from build123d import *

# Parameters (mm, degrees)
ESQUISSE1_W             = 40
ESQUISSE1_H             = 40
BOSS_EXTRU_1_DEPTH      = 30
ENL_V_MAT_EXTRU_1_DEPTH = 30
ESQUISSE4_R             = 1.5
ENL_V_MAT_EXTRU_2_DEPTH = 41
ESQUISSE5_R             = 1.5
ENL_V_MAT_EXTRU_3_DEPTH = 41
ESQUISSE6_W             = 23
ESQUISSE6_H             = 27
ESQUISSE6_H_2           = 20.20636544
ESQUISSE6_H_3           = 20.206365439
BOSS_EXTRU_2_DEPTH      = 10
ESQUISSE7_R             = 3
ENL_V_MAT_EXTRU_4_DEPTH = 11.0000001


with BuildPart() as part:
    # Esquisse1 → Boss.-Extru.1 (new body)
    with BuildSketch(Plane.XY):
        with Locations((0, 559.576541314)):
            Rectangle(ESQUISSE1_W, ESQUISSE1_H)
        with BuildLine():
            Line((-10.025728158, 549.777097393), (9.970271386, 549.3770946))
            Line((9.970271386, 549.3770946), (9.998865294, 550.806494043))
            ThreePointArc((9.998865294, 550.806494043), (9.591165544, 551.864859717), (8.559153746, 552.335294236))
            Line((8.559153746, 552.335294236), (4.551996141, 552.495677906))
            ThreePointArc((4.551996141, 552.495677906), (2.508650242, 553.414808545), (1.671972976, 555.493277873))
            Line((1.671972976, 555.493277873), (1.671972976, 568.566900265))
            ThreePointArc((1.671972976, 568.566900265), (1.386115868, 569.266900215), (0.691973116, 569.566700242))
            Line((0.691973116, 569.566700242), (0.052575697, 569.579490838))
            ThreePointArc((0.052575697, 569.579490838), (-0.653001419, 569.307691005), (-0.966624431, 568.619683139))
            Line((-0.966624431, 568.619683139), (-1.489468376, 555.556519791))
            ThreePointArc((-1.489468376, 555.556519791), (-2.408599014, 553.513173892), (-4.487068342, 552.676496626))
            Line((-4.487068342, 552.676496626), (-8.497434284, 552.676496626))
            ThreePointArc((-8.497434284, 552.676496626), (-9.54743421, 552.247710964), (-9.99713425, 551.206496835))
            Line((-9.99713425, 551.206496835), (-10.025728158, 549.777097393))
        make_face(mode=Mode.SUBTRACT)
    extrude(amount=BOSS_EXTRU_1_DEPTH)

    # Esquisse3 → Enlèv. mat.-Extru.1 (cut)
    with BuildSketch(Plane.XY.offset(30)):
        with BuildLine():
            Line((0.701973186, 570.066600231), (0.062575767, 570.079390827))
            ThreePointArc((0.062575767, 570.079390827), (-0.995789907, 569.671691077), (-1.466224425, 568.639679279))
            Line((-1.466224425, 568.639679279), (-1.98906837, 555.57651593))
            ThreePointArc((-1.98906837, 555.57651593), (-2.755010569, 553.873727681), (-4.487068342, 553.176496626))
            Line((-4.487068342, 553.176496626), (-8.497434284, 553.176496626))
            ThreePointArc((-8.497434284, 553.176496626), (-9.897434185, 552.604782409), (-10.497034239, 551.216496905))
            Line((-10.497034239, 551.216496905), (-10.535628216, 549.287197474))
            Line((-10.535628216, 549.287197474), (10.460171305, 548.867194542))
            Line((10.460171305, 548.867194542), (10.498765283, 550.796493973))
            ThreePointArc((10.498765283, 550.796493973), (9.955165615, 552.207648206), (8.579149885, 552.83489423))
            Line((8.579149885, 552.83489423), (4.57199228, 552.995277901))
            ThreePointArc((4.57199228, 552.995277901), (2.869204031, 553.761220099), (2.171972976, 555.493277873))
            Line((2.171972976, 555.493277873), (2.171972976, 568.566900265))
            ThreePointArc((2.171972976, 568.566900265), (1.743187314, 569.61690019), (0.701973186, 570.066600231))
        make_face()
    extrude(amount=-ENL_V_MAT_EXTRU_1_DEPTH, mode=Mode.SUBTRACT)

    # Esquisse4 → Enlèv. mat.-Extru.2 (cut, through all)
    with BuildSketch(Plane.XZ.offset(-539.576541314)):
        with Locations(Location((-6.523433168, 24.203853726, 0), (0, 0, 270))):  # turned: the seam where the file's is
            Circle(ESQUISSE4_R)
        with Locations(Location((-6.523433168, 5.901559872, 0), (0, 0, 270))):  # turned: the seam where the file's is
            Circle(ESQUISSE4_R)
        with Locations((7.005369476, 5.612158233)):
            Circle(ESQUISSE4_R)
        with Locations((7.788039062, 23.897709596)):
            Circle(ESQUISSE4_R)
    extrude(amount=-ENL_V_MAT_EXTRU_2_DEPTH, mode=Mode.SUBTRACT)

    # Esquisse5 → Enlèv. mat.-Extru.3 (cut, through all)
    with BuildSketch(Plane.ZY.offset(20)):
        with Locations(Location((27.786828978, 562.049365696, 0), (0, 0, 270))):  # turned: the seam where the file's is
            Circle(ESQUISSE5_R)
        with Locations(Location((2.00094519, 562.049365696, 0), (0, 0, 270))):  # turned: the seam where the file's is
            Circle(ESQUISSE5_R)
    extrude(amount=-ENL_V_MAT_EXTRU_3_DEPTH, mode=Mode.SUBTRACT)

    # Esquisse6 → Boss.-Extru.2 (add)
    with BuildSketch(Plane(origin=(0, 0, 0), x_dir=(-1, 0, 0), z_dir=(0, 0, -1))):
        with Locations((-23.5, 581.076541314)):
            Rectangle(ESQUISSE6_W, ESQUISSE6_H)
        with Locations((22.166061681, 537.286666725)):
            Rectangle(ESQUISSE6_W, ESQUISSE6_H_2)
        with Locations((21.063566891, 581.241581079)):
            Rectangle(ESQUISSE6_W, ESQUISSE6_H)
        with Locations((-23.306010365, 536.648365215)):
            Rectangle(ESQUISSE6_W, ESQUISSE6_H_3)
    extrude(amount=-BOSS_EXTRU_2_DEPTH)

    # Esquisse7 → Enlèv. mat.-Extru.4 (cut, through all)
    with BuildSketch(Plane.XY.offset(10)):
        with Locations((-27.359707791, 589.516341352)):
            Circle(ESQUISSE7_R)
        with Locations((-27.359707791, 573.664786381)):
            Circle(ESQUISSE7_R)
        with Locations((-27.359707791, 541.773153337)):
            Circle(ESQUISSE7_R)
        with Locations((-27.359707791, 531.883070045)):
            Circle(ESQUISSE7_R)
        with Locations((-17.338422342, 531.883070045)):
            Circle(ESQUISSE7_R)
        with Locations((-17.338422342, 589.516341352)):
            Circle(ESQUISSE7_R)
        with Locations((17.587577233, 589.516341352)):
            Circle(ESQUISSE7_R)
        with Locations((29.13602426, 589.516341352)):
            Circle(ESQUISSE7_R)
        with Locations((29.13602426, 573.664786381)):
            Circle(ESQUISSE7_R)
        with Locations((29.13602426, 541.773153337)):
            Circle(ESQUISSE7_R)
        with Locations((29.13602426, 531.883070045)):
            Circle(ESQUISSE7_R)
        with Locations((17.587577233, 531.883070045)):
            Circle(ESQUISSE7_R)
    extrude(amount=-ENL_V_MAT_EXTRU_4_DEPTH, mode=Mode.SUBTRACT)


solid = part.part
The listing builds one solid part. Answer for the finished solid, in the listing's coordinates (mm). A direction names the side the tool comes from. Coordinates: 2 decimals unless noted, no trailing zeros. Write each loop counter-clockwise with the first axis right and the second up, starting at its lowest first coordinate (ties: lowest second). Pieces come first, ordered by that corner, then holes. Notation, with made-up numbers: M -4.75,43.25 L 21.25,43.25 A31 ccw 21.25,82.25 Z; hole C -19.75,2.5 d4. An arc over 180 degrees is marked long. Write each question's results on one line, items separated by ' | '.
Item 1: The part is cut by section D-D on x = 30. Determine the outline of the cut face in (y, z).
Answer below:
outline: M 526.55,0 L 529.01,0 L 529.01,10 L 526.55,10 Z; M 534.76,0 L 538.9,0 L 538.9,10 L 534.76,10 Z; M 544.65,0 L 546.75,0 L 546.75,10 L 544.65,10 Z; M 567.58,0 L 570.79,0 L 570.79,10 L 567.58,10 Z; M 576.54,0 L 586.64,0 L 586.64,10 L 576.54,10 Z; M 592.39,0 L 594.58,0 L 594.58,10 L 592.39,10 Z
Item 2: The part is cut by section C-C on y = 575. Determine the outline of the cut face in (x, z), and give its area (3 significant figures).
Answer below:
outline: M -32.56,0 L -30.05,0 L -30.05,10 L -32.56,10 Z; M -24.67,0 L 26.45,0 L 26.45,10 L 20,10 L 20,30 L -20,30 L -20,10 L -24.67,10 Z; M 31.82,0 L 35,0 L 35,10 L 31.82,10 Z; hole C -6.52,5.9 d3; hole C -6.52,24.2 d3; hole C 7.01,5.61 d3; hole C 7.79,23.9 d3 | area: 1,340 mm2
Item 3: Given P1, Ø15, axis at x = 1.5, z = 16.5, coming from the -Y side; P2, Ø5, axis at x = -23.5, z = 7, coming from the -Y side; P3, Ø2, axis at y = 581, z = 6, coming from the -X side, each flat-ended and moving along its own axis, determine where each tip first touches the part or whether it passes through.
Answer below:
P1: y = 539.58 | P2: y = 527.18 | P3: x = -32.56
Item 4: Which of the six approach directions +Z, -Z, +X, -X, +Y, -Y give full straight-line access (tool end or side, diameter ignored) to faces 4 (the face through (12, 587, 5)), 5 (the face through (6.68, 565.94, 24.91)), 6 (the face through (6.604, 552.914, 15.21))?
Answer below:
face 4: +Z, -Z, +Y | face 5: +Y, -Y | face 6: +Z, -Z
Item 5: For a pull along Y with two mould halves and no side action, classify faces 1 (the face through (-20, 559, 18)), 2 (the face through (-22, 527.183, 5)), 3 (the face through (-5, 560, 30)) as released by +Y, released by -Y, zero draft, split by the parting line, or undercut.
Answer below:
face 1: undercut | face 2: released by -Y | face 3: zero draft
Item 6: The part is cut by section B-B on z = 20.5. Determine the outline of the cut face in (x, y).
Answer below:
outline: M -20,539.58 L 20,539.58 L 20,579.58 L -20,579.58 Z; hole M -10.54,549.29 L 10.46,548.87 L 10.5,550.8 A2 ccw 8.58,552.83 L 4.57,553 A2.5 cw 2.17,555.49 L 2.17,568.57 A1.5 ccw 0.7,570.07 L 0.06,570.08 A1.5 ccw -1.47,568.64 L -1.99,555.58 A2.5 cw -4.49,553.18 L -8.5,553.18 A2 ccw -10.5,551.22 Z
Item 7: The part is cut by section A-A on y = 585. Determine the outline of the cut face in (x, z).
Answer below:
outline: M -32.56,0 L -9.56,0 L -9.56,10 L -32.56,10 Z; M 12,0 L 35,0 L 35,10 L 12,10 Z
Item 8: Consider probe 1 along X at (y, z) = (571, 24); probe 2 along X at (y, z) = (537.5, 8.5); probe 3 along X at (y, z) = (558.5, 5.5). Determine where each line is inside the solid, lowest interval first. Write a range as [from, to].
Answer below:
probe 1: [-20, -8.01], [-5.04, 6.29], [9.28, 20] | probe 2: [-33.67, -10.67], [11.81, 34.81] | probe 3: [-20, -7.97], [-5.08, -1.87], [2.17, 5.51], [8.5, 20]
